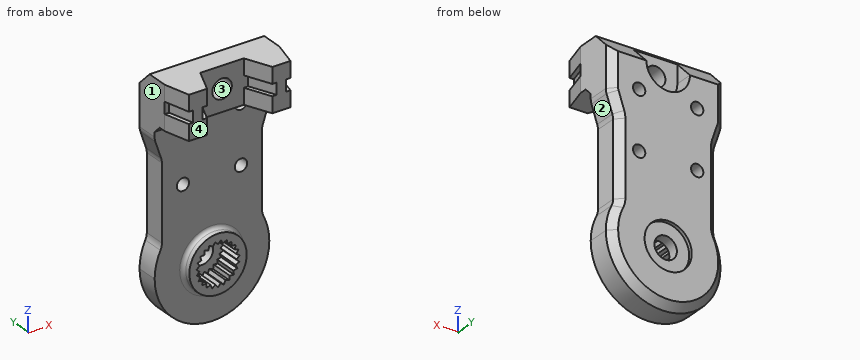
```python
from build123d import *
from build123d.topology import SkipClean

# Parameters (mm, degrees)
EXTRUDE_1_DEPTH          = 4
EXTRUDE_3_DEPTH          = 6
CHAMFER_1_SIZE           = 3
SKETCH_5_R               = 0.85
CUT_EXTRUDE_1_DEPTH      = 4
PATTERN_LINEAR_1_COUNT   = 2
PATTERN_LINEAR_1_PITCH   = 8
CUT_EXTRUDE_2_DEPTH      = 2.5
CUT_EXTRUDE_3_REACH      = 30.061
SKETCH_7_R               = 1.35
SKETCH_8_R               = 3.95
EXTRUDE_4_DEPTH          = 1.2
SKETCH_9_R               = 3.25
CUT_EXTRUDE_4_DEPTH      = 0.5
SKETCH_10_R              = 1.55
CUT_EXTRUDE_5_DEPTH      = 29.786455148
FILLET_1_R               = 0.5
SKETCH_11_R              = 3
CUT_EXTRUDE_6_DEPTH      = 3.2
EXTRUDE_5_DEPTH          = 3.2
PATTERN_CIRCULAR_1_COUNT = 23
CUT_EXTRUDE_7_DEPTH      = 0.8
CUT_EXTRUDE_8_DEPTH      = 29.786455148
FILLET_2_R               = 2
CHAMFER_2_SIZE           = 1


with BuildPart() as part:
    # ｽｹｯﾁ1 → ﾎﾞｽ - 押し出し1 (new body)
    with BuildSketch(Plane(origin=(0, 0, 0), x_dir=(1, 0, 0), z_dir=(0, 1, 0))):
        with BuildLine():
            Line((-7.9, 0), (-7.9, -26))
            Line((-7.9, -26), (7.9, -26))
            Line((7.9, -26), (7.9, 0))
            ThreePointArc((7.9, 0), (0, 7.9), (-7.9, 0))
        make_face()
    extrude(amount=EXTRUDE_1_DEPTH)

    # ｽｹｯﾁ4 → ﾎﾞｽ - 押し出し3 (add)
    with BuildSketch(Plane.XY.offset(26)):
        Polygon((-7, -5.5), (-4.5, -5.5), (-3, -2), (3, -2), (4.5, -5.5), (7, -5.5), (7.9, -2), (7.9, 0), (-7.9, 0), (-7.9, -2), align=None)
    extrude(amount=-EXTRUDE_3_DEPTH)

    # 面取り1
    chamfer_1_edges = [part.edges().sort_by_distance(p)[0] for p in [
        (0, 4, 26),
    ]]
    chamfer(chamfer_1_edges, length=CHAMFER_1_SIZE)

    # ｽｹｯﾁ5 → ｶｯﾄ - 押し出し1 (cut)
    with BuildSketch(Plane(origin=(0, 4, 0), x_dir=(1, 0, 0), z_dir=(0, 1, 0))):
        with Locations(Location((-4, -19, 0), (0, 0, 270))):
            Circle(SKETCH_5_R)
        with Locations(Location((4, -19, 0), (0, 0, 270))):
            Circle(SKETCH_5_R)
    cut_extrude_1 = extrude(amount=-CUT_EXTRUDE_1_DEPTH, mode=Mode.SUBTRACT)

    # 直線ﾊﾟﾀｰﾝ1: ｶｯﾄ - 押し出し1 ×2
    with Locations(*[(0, 0, -i * PATTERN_LINEAR_1_PITCH) for i in range(1, PATTERN_LINEAR_1_COUNT)]):
        add(cut_extrude_1, mode=Mode.SUBTRACT)

    # ｽｹｯﾁ6 → ｶｯﾄ - 押し出し2 (cut)
    with BuildSketch(Plane(origin=(0, 4, 0), x_dir=(1, 0, 0), z_dir=(0, 1, 0))):
        with BuildLine():
            Line((-3, -23), (-3, -27))
            Line((-3, -27), (3, -27))
            Line((3, -27), (3, -23))
            ThreePointArc((3, -23), (0, -20), (-3, -23))
        make_face()
    extrude(amount=-CUT_EXTRUDE_2_DEPTH, mode=Mode.SUBTRACT)

    # ｽｹｯﾁ7 → ｶｯﾄ - 押し出し3 (cut, up to next)
    with BuildSketch(Plane(origin=(0, 1.5, 0), x_dir=(1, 0, 0), z_dir=(0, 1, 0)), mode=Mode.PRIVATE) as cut_extrude_3_sk1:
        with Locations(Location((0, -23, 0), (0, 0, 270))):
            Circle(SKETCH_7_R)
    cut_extrude_3_tool1 = extrude(cut_extrude_3_sk1.sketch, amount=-CUT_EXTRUDE_3_REACH, mode=Mode.PRIVATE) & part.part
    add(cut_extrude_3_tool1.solids().sort_by_distance((0, 1.5, 23))[0], mode=Mode.SUBTRACT)

    # ｽｹｯﾁ8 → ﾎﾞｽ - 押し出し4 (add)
    with BuildSketch(Plane.XZ):
        with Locations(Location((0, 0, 0), (0, 0, 90))):
            Circle(SKETCH_8_R)
    extrude(amount=EXTRUDE_4_DEPTH)

    # ｽｹｯﾁ9 → ｶｯﾄ - 押し出し4 (cut)
    with BuildSketch(Plane(origin=(0, 4, 0), x_dir=(1, 0, 0), z_dir=(0, 1, 0))):
        with Locations(Location((0, 0, 0), (0, 0, 270))):
            Circle(SKETCH_9_R)
    extrude(amount=-CUT_EXTRUDE_4_DEPTH, mode=Mode.SUBTRACT)

    # ｽｹｯﾁ10 → ｶｯﾄ - 押し出し5 (cut, through all)
    with BuildSketch(Plane(origin=(0, 4, 0), x_dir=(1, 0, 0), z_dir=(0, 1, 0))):
        with Locations(Location((0, 0, 0), (0, 0, 270))):
            Circle(SKETCH_10_R)
    extrude(amount=-CUT_EXTRUDE_5_DEPTH, mode=Mode.SUBTRACT)

    # ﾌｨﾚｯﾄ1
    fillet_1_edges = [part.edges().sort_by_distance(p)[0] for p in [
        (0, 0, -3.95),
    ]]
    fillet(fillet_1_edges, radius=FILLET_1_R)

    # ｽｹｯﾁ11 → ｶｯﾄ - 押し出し6 (cut)
    with BuildSketch(Plane.XZ.offset(1.2)):
        with Locations(Location((0, 0, 0), (0, 0, 270))):
            Circle(SKETCH_11_R)
    extrude(amount=-CUT_EXTRUDE_6_DEPTH, mode=Mode.SUBTRACT)

    # ｽｹｯﾁ12 → ﾎﾞｽ - 押し出し5 (add)
    with BuildSketch(Plane.XZ.offset(1.2)):
        with BuildLine():
            Line((-0.408499947, 2.972057838), (0, 2.574530741))
            Line((0, 2.574530741), (0.408499947, 2.972057838))
            ThreePointArc((0.408499947, 2.972057838), (0, 3), (-0.408499947, 2.972057838))
        make_face()
    extrude_5 = extrude(amount=-EXTRUDE_5_DEPTH)

    # 円形ﾊﾟﾀｰﾝ1: ﾎﾞｽ - 押し出し5 ×23 about axis
    pattern_circular_1_axis = Axis((0, 0, 0), (0, 1, 0))
    for i in range(1, PATTERN_CIRCULAR_1_COUNT):
        add(extrude_5.rotate(pattern_circular_1_axis, i * 360 / PATTERN_CIRCULAR_1_COUNT))

    # ｽｹｯﾁ13 → ｶｯﾄ - 押し出し7 (cut, symmetric)
    with BuildSketch(Plane.XY.offset(23)):
        Polygon((3, -2), (4.5, -5.5), (5.1, -5.5), (3.6, -2), align=None)
        Polygon((7.9, -2), (7, -5.5), (6.4, -5.5), (7.3, -2), align=None)
    cut_extrude_7 = extrude(amount=CUT_EXTRUDE_7_DEPTH, both=True, mode=Mode.SUBTRACT)

    # ﾐﾗｰ1: ｶｯﾄ - 押し出し7 across plane
    add(cut_extrude_7.mirror(Plane(origin=(0, 0, 0), x_dir=(0, 0, 1), z_dir=(1, 0, 0))), mode=Mode.SUBTRACT)

    # ｽｹｯﾁ14 → ｶｯﾄ - 押し出し8 (cut, through all)
    with SkipClean():  # the faces are left unmerged after this step: merging them gives an invalid solid
        with BuildSketch(Plane(origin=(0, 4, 0), x_dir=(1, 0, 0), z_dir=(0, 1, 0))):
            with BuildLine():
                Line((-7.9, 0), (-7.9, -18))
                Line((-7.9, -18), (-6.9, -15))
                Line((-6.9, -15), (-6.9, -3.847076812))
                ThreePointArc((-6.9, -3.847076812), (-7.645913941, -1.987460691), (-7.9, 0))
            make_face()
        cut_extrude_8 = extrude(amount=-CUT_EXTRUDE_8_DEPTH, mode=Mode.SUBTRACT)

    # ﾐﾗｰ2: ｶｯﾄ - 押し出し8 across plane
    with SkipClean():  # the faces are left unmerged after this step: merging them gives an invalid solid
        add(cut_extrude_8.mirror(Plane(origin=(0, 0, 0), x_dir=(0, 0, 1), z_dir=(1, 0, 0))), mode=Mode.SUBTRACT)

    # ﾌｨﾚｯﾄ2
    fillet_2_edges = [part.edges().sort_by_distance(p)[0] for p in [
        (-6.9, 2, 3.847076812),
        (-6.9, 2, 15),
        (-7.9, 2, 18),
        (6.9, 2, 3.847076812),
        (7.9, 2, 18),
        (6.9, 2, 15),
    ]]
    fillet(fillet_2_edges, radius=FILLET_2_R)

    # 面取り2
    # the kernel refuses this chamfer: 1 mm, written as the material it adds along each edge
    with BuildSketch(Plane(origin=(7.9, 0, 20), x_dir=(0, 0.02749587661058639, -0.9996219169112968), z_dir=(-1, 0, 0))) as chamfer_2_piece_1_section:
        Polygon((CHAMFER_2_SIZE * 0.999621916911, CHAMFER_2_SIZE * 0.0274958766106), (-CHAMFER_2_SIZE * 0.0274958766106, CHAMFER_2_SIZE * 0.999621916911), (0, 0), align=None)
    chamfer_2_piece_1 = extrude(amount=15.8, mode=Mode.PRIVATE)
    chamfer_2_piece_1 = chamfer_2_piece_1 - Plane(origin=(-4, -0.34097177, 19), x_dir=(0, 0, 1), z_dir=(0, 1, 0)) * Cylinder(0.85, 36, mode=Mode.PRIVATE)
    chamfer_2_piece_1 = chamfer_2_piece_1 - Plane(origin=(4, -0.34097177, 19), x_dir=(0, 0, 1), z_dir=(0, 1, 0)) * Cylinder(0.85, 36, mode=Mode.PRIVATE)
    add(chamfer_2_piece_1)
    # the kernel refuses this chamfer: 1 mm, written as the material it takes off along each edge
    with BuildSketch(Plane(origin=(-7.9, 4, 18.32455532), x_dir=(-0.027495876610586487, -0.9996219169112968, 0), z_dir=(0, 0, 1)), Plane(origin=(7.9, 4, 25.571682988), x_dir=(0.027495876610586487, -0.9996219169112968, 0), z_dir=(0, 0, -1))) as chamfer_2_2_piece_1:
        Polygon((CHAMFER_2_SIZE * 0.999621916911, CHAMFER_2_SIZE * 0.0274958766106), (-CHAMFER_2_SIZE * 0.0274958766106, CHAMFER_2_SIZE * 0.999621916911), (0, 0), align=None)
    extrude(amount=7.247127668, mode=Mode.SUBTRACT)
    with BuildSketch(Plane(origin=(0, 4, 0), x_dir=(1, 0, 0), z_dir=(0, 0, 1))) as chamfer_2_2_piece_2:
        Polygon((7.9, -CHAMFER_2_SIZE), (7.9 - CHAMFER_2_SIZE, 0), (7.9, 0), align=None)
    revolve(axis=Axis((0, 4, 0), (0, 1, 0)), revolution_arc=180, mode=Mode.SUBTRACT)
    with BuildSketch(Plane(origin=(-5.9, 4, 18.32455532), x_dir=(-1, 0, 0), z_dir=(0, 0, 1))) as chamfer_2_2_piece_3:
        Polygon((2, CHAMFER_2_SIZE), (2 - CHAMFER_2_SIZE, 0), (2, 0), align=None)
    revolve(axis=Axis((-5.9, 4, 18.32455532), (0, -1, 0)), revolution_arc=18.434948823, mode=Mode.SUBTRACT)
    with BuildSketch(Plane(origin=(-7.797366596, 4, 17.692099788), x_dir=(-0.026084878905721698, -0.9996219169112968, -0.008694959635240574), z_dir=(0.3162277660168382, 0, -0.9486832980505138))) as chamfer_2_2_piece_4:
        Polygon((CHAMFER_2_SIZE * 0.999621916911, -CHAMFER_2_SIZE * 0.0274958766106), (-CHAMFER_2_SIZE * 0.0274958766106, -CHAMFER_2_SIZE * 0.999621916911), (0, 0), align=None)
    extrude(amount=2.513167019, mode=Mode.SUBTRACT)
    with BuildSketch(Plane(origin=(-8.9, 4, 14.67544468), x_dir=(0.9486832980505138, 0, 0.31622776601683794), z_dir=(-0.31622776601683794, 0, 0.9486832980505138))) as chamfer_2_2_piece_5:
        Polygon((2, -CHAMFER_2_SIZE), (2 + CHAMFER_2_SIZE, 0), (2, 0), align=None)
    revolve(axis=Axis((-8.9, 4, 14.67544468), (0, 1, 0)), revolution_arc=18.434948823, mode=Mode.SUBTRACT)
    with BuildSketch(Plane(origin=(-6.9, 4, 14.67544468), x_dir=(-0.027495876610586487, -0.9996219169112968, 0), z_dir=(0, 0, -1))) as chamfer_2_2_piece_6:
        Polygon((CHAMFER_2_SIZE * 0.999621916911, -CHAMFER_2_SIZE * 0.0274958766106), (-CHAMFER_2_SIZE * 0.0274958766106, -CHAMFER_2_SIZE * 0.999621916911), (0, 0), align=None)
    extrude(amount=10.339548002, mode=Mode.SUBTRACT)
    with BuildSketch(Plane(origin=(-8.9, 4, 4.335896678), x_dir=(1, 0, 0), z_dir=(0, 0, 1))) as chamfer_2_2_piece_7:
        Polygon((2, -CHAMFER_2_SIZE), (2 + CHAMFER_2_SIZE, 0), (2, 0), align=None)
    revolve(axis=Axis((-8.9, 4, 4.335896678), (0, 1, 0)), revolution_arc=25.974390018, mode=Mode.SUBTRACT)
    with BuildSketch(Plane(origin=(8.9, 4, 4.335896678), x_dir=(-0.8989898989898986, 0, -0.43796936138745124), z_dir=(0.43796936138745124, 0, -0.8989898989898986))) as chamfer_2_2_piece_8:
        Polygon((2, -CHAMFER_2_SIZE), (2 + CHAMFER_2_SIZE, 0), (2, 0), align=None)
    revolve(axis=Axis((8.9, 4, 4.335896678), (0, 1, 0)), revolution_arc=25.974390018, mode=Mode.SUBTRACT)
    with BuildSketch(Plane(origin=(6.9, 4, 14.67544468), x_dir=(0.027495876610586487, -0.9996219169112968, 0), z_dir=(0, 0, -1))) as chamfer_2_2_piece_9:
        Polygon((CHAMFER_2_SIZE * 0.999621916911, CHAMFER_2_SIZE * 0.0274958766106), (-CHAMFER_2_SIZE * 0.0274958766106, CHAMFER_2_SIZE * 0.999621916911), (0, 0), align=None)
    extrude(amount=10.339548002, mode=Mode.SUBTRACT)
    with BuildSketch(Plane(origin=(8.9, 4, 14.67544468), x_dir=(-1, 0, 0), z_dir=(0, 0, -1))) as chamfer_2_2_piece_10:
        Polygon((2, -CHAMFER_2_SIZE), (2 + CHAMFER_2_SIZE, 0), (2, 0), align=None)
    revolve(axis=Axis((8.9, 4, 14.67544468), (0, 1, 0)), revolution_arc=18.434948823, mode=Mode.SUBTRACT)
    with BuildSketch(Plane(origin=(7.797366596, 4, 17.692099788), x_dir=(0.02608487890572092, -0.9996219169112968, -0.008694959635240314), z_dir=(-0.3162277660168382, 0, -0.9486832980505138))) as chamfer_2_2_piece_11:
        Polygon((CHAMFER_2_SIZE * 0.999621916911, CHAMFER_2_SIZE * 0.0274958766106), (-CHAMFER_2_SIZE * 0.0274958766106, CHAMFER_2_SIZE * 0.999621916911), (0, 0), align=None)
    extrude(amount=2.513167019, mode=Mode.SUBTRACT)
    with BuildSketch(Plane(origin=(5.9, 4, 18.32455532), x_dir=(0.9486832980505135, 0, -0.3162277660168389), z_dir=(-0.3162277660168389, 0, -0.9486832980505135))) as chamfer_2_2_piece_12:
        Polygon((2, CHAMFER_2_SIZE), (2 - CHAMFER_2_SIZE, 0), (2, 0), align=None)
    revolve(axis=Axis((5.9, 4, 18.32455532), (0, -1, 0)), revolution_arc=18.434948823, mode=Mode.SUBTRACT)
    with BuildSketch(Plane(origin=(0, 4, 0), x_dir=(0.8989898989898988, 0, 0.43796936138745096), z_dir=(-0.43796936138745096, 0, 0.8989898989898988))) as chamfer_2_2_piece_13:
        Polygon((7.9, -CHAMFER_2_SIZE), (7.9 - CHAMFER_2_SIZE, 0), (7.9, 0), align=None)
    revolve(axis=Axis((0, 4, 0), (0, 1, 0)), revolution_arc=25.974390018, mode=Mode.SUBTRACT)
    with BuildSketch(Plane(origin=(0, 4, 0), x_dir=(-0.8989898989898988, 0, 0.43796936138745096), z_dir=(0.43796936138745096, 0, 0.8989898989898988))) as chamfer_2_2_piece_14:
        Polygon((7.9, CHAMFER_2_SIZE), (7.9 - CHAMFER_2_SIZE, 0), (7.9, 0), align=None)
    revolve(axis=Axis((0, 4, 0), (0, -1, 0)), revolution_arc=25.974390018, mode=Mode.SUBTRACT)


solid = part.part
```
Model file for the job. Use its own axes, mm. Face numbers are marked on the shaded views. Coordinates: 2 decimals unless noted, no trailing zeros. Loops run counter-clockwise (first coordinate to the right, second up) from the corner with the lowest first, then second, coordinate; pieces in that order, holes last. Notation, with made-up numbers: (33.25, 27) -> (60.25, 27) arc R31 ccw to (60.25, 53) -> close; hole circle Ø4 at (-15.5, -17.5). An arc over 180 degrees is marked (long way). Answer as a JSON object with one key per item and string values.
Q1. Cut at D-D (y = 0.5). State how many separate pieces and enclosed holes the cut face has, and give its area (3 significant figures).
Report:
{"separate pieces": "1", "enclosed holes": "6", "area": "442 mm2"}
Q2. Flat gauge pins, fed straight in: P1, Ø2, axis at x = 6, z = 12.5, coming from the +Y side; P2, Ø3.5, axis at x = 0, z = 23, coming from the -Y side; P3, Ø5, axis at x = -5.5, y = 1, coming from the -Z side; P4, Ø6.5, axis at x = 1, z = -1.5, coming from the -Y side. Where does each tip first touch, or does it go through?
Report:
{"P1": "stops at y = 4", "P2": "stops at y = -2", "P3": "stops at z = -7.31", "P4": "stops at y = -1.2"}
Q3. Cut at B-B (z = 11). List the corners of the cut face in (x, y), and give its area (3 significant figures).
Report:
{"outline": "(-6.9, 0) -> (-4.85, 0) -> (-4.85, 4) -> (-5.9, 4) -> (-6.9, 3) -> close; (-3.15, 0) -> (3.15, 0) -> (3.15, 4) -> (-3.15, 4) -> close; (4.85, 0) -> (6.9, 0) -> (6.9, 3) -> (5.9, 4) -> (4.85, 4) -> close", "area": "40.6 mm2"}
Q4. Cut at A-A (y = -3.75). List the corners of the cut face in (x, z).
Report:
{"outline": "(-7.45, 20) -> (-3.75, 20) -> (-3.75, 22.2) -> (-4.35, 22.2) -> (-4.35, 23.8) -> (-3.75, 23.8) -> (-3.75, 26) -> (-7.45, 26) -> (-7.45, 23.8) -> (-6.85, 23.8) -> (-6.85, 22.2) -> (-7.45, 22.2) -> close; (3.75, 20) -> (7.45, 20) -> (7.45, 22.2) -> (6.85, 22.2) -> (6.85, 23.8) -> (7.45, 23.8) -> (7.45, 26) -> (3.75, 26) -> (3.75, 23.8) -> (4.35, 23.8) -> (4.35, 22.2) -> (3.75, 22.2) -> close"}
Q5. Probe probe 1 along X at (y, z) = (2.6, 19); probe 2 along X at (y, z) = (2.2, 11); probe 3 along X at (y, z) = (-0.5, 23). List the from-to ranges inside material, lowest first.
Report:
{"probe 1": "x = -7.9 to -4.85, -3.15 to 3.15, 4.85 to 7.9", "probe 2": "x = -6.9 to -4.85, -3.15 to 3.15, 4.85 to 6.9", "probe 3": "x = -7.9 to -1.35, 1.35 to 7.9"}
Q6. Cut at C-C (z = 5). List the corners of the cut face in (x, y).
Report:
{"outline": "(-6.9, 0) -> (6.9, 0) -> (6.9, 3) -> (5.9, 4) -> (-5.9, 4) -> (-6.9, 3) -> close"}
Q7. Pull direction X, two halves, no side cores. Call the marked faces 1, 2, 3 and 4: released by +X, released by -X, zero draft, split by the parting line, or undercut.
Report:
{"face 1": "released by -X", "face 2": "released by +X", "face 3": "undercut", "face 4": "zero draft"}
